Geometry: final body of the model. Coordinates: model frame, mm. A direction names the side the tool comes from. Give positions to 0.01 mm unless a question says otherwise; leave off trailing zeros. Write each loop counter-clockwise with the first axis right and the second up, starting at its lowest first coordinate (ties: lowest second). Pieces come first, ordered by that corner, then holes. Notation, with made-up numbers: (47, -36.5) -> (64, -36.5) arc R18 ccw to (64, -24.5) -> close; hole circle Ø6 at (32.5, 82.25). An arc over 180 degrees is marked (long way). Answer in a Markdown table with one row per item. Add a question column.
Item 1: Draft query along Z for faces 4 (the flat face through (350.266, 55, 187)), 5 (the flat face through (181.824, 28.354, 12.186)), 6 (the flat face through (182, 180, 0)), 7 (the flat face through (368.3, 213, 195)). Return one class per face: +Z half, -Z half, draft (parallel to the pull), parting line (faces both ways), or undercut.
Item 2: Section query B-B on y = 150. Output: boundary loops of the cut face in (x, z).
Item 3: Access query for faces 1 (the flat face through (181.824, 56.286, 19.184)), 2 (the flat face through (181.57, 397.83, 151.55)), 3 (the flat face through (181.82, 93.53, 364.05)). Directions: +Z, -Z, +X, -X, +Y, -Y. A direction counts if a zero-diameter tool reaches every point of the face in a straight line with its end or side. Return the directions, or none.
Item 4: First-contact query: P1, Ø5, axis at x = 274.5, z = 233, coming from the +Y side; P2, Ø8, axis at x = 277, z = 103, coming from the +Y side; P3, Ø1.5, axis at x = 294, y = 175, coming from the +Z side. Flat tips, straight axial feed; report the tip coordinate or a pass-through.
Item 5: Material intervals for probe 1 along X at (y, z) = (45, 133); probe 2 along Z at (x, y) = (68.5, 165); probe 3 along Z at (x, y) = (237.5, 21.5), sorted ascending. Write a range as from..to.
Item 6: Section query C-C on x = 191.5. Output: boundary loops of the cut face in (y, z).
Item 7: Section query A-A on x = 237. Output: boundary loops of the cut face in (y, z).
Item 8: Section query D-D on y = 296. Output: boundary loops of the cut face in (x, z), plus the area to 3 significant figures.
```python
from build123d import *

# Parameters (mm, degrees)
F1_DEPTH = 368.3
F2_W     = 332.232
F2_H     = 357.632
F3_DEPTH = 25.4
F4_R     = 130.175
F5_DEPTH = 10.16
F6_W     = 332.232
F6_H     = 25.4
F7_DEPTH = 25.4


with BuildPart() as f1:
    # F0 (on Right) → F1 (new body)
    with BuildSketch(Plane.YZ):
        Polygon((85.2122760074, 384.3677380031), (0, 0), (364.2337952902, 0), (432.3831361393, 307.4018112867), align=None)
    extrude(amount=F1_DEPTH)

    # F2 (on face) → F3 (cut)
    with BuildSketch(Plane(origin=(0, 0, 0), x_dir=(1, 0, 0), z_dir=(0, -0.9762960071, 0.2164396139))):
        with Locations((184.15, 196.85)):
            Rectangle(F2_W, F2_H)
    extrude(amount=-F3_DEPTH, mode=Mode.SUBTRACT)

    # F4 (on face) → F5 (join)
    with BuildSketch(Plane(origin=(0, 24.7979185808, -5.497566194), x_dir=(1, 0, 0), z_dir=(0, -0.9762960071, 0.2164396139))):
        with Locations((184.15, 210.566)):
            Circle(F4_R)
    extrude(amount=F5_DEPTH)

    # F6 (on face) → F7 (cut)
    with BuildSketch(Plane(origin=(0, 24.7979185808, -5.497566194), x_dir=(1, 0, 0), z_dir=(0, -0.9762960071, 0.2164396139))):
        with Locations((184.15, 30.734)):
            Rectangle(F6_W, F6_H)
    extrude(amount=-F7_DEPTH, mode=Mode.SUBTRACT)


solid = f1.part
```
Findings below:
| question | item | result |
|---|---|---|
| 1 | face 4 | undercut |
| 1 | face 5 | undercut |
| 1 | face 6 | -Z half |
| 1 | face 7 | draft |
| 2 | outline | (0, 0) -> (368.3, 0) -> (368.3, 370) -> (0, 370) -> close |
| 3 | face 1 | none |
| 3 | face 2 | -Z, +X, -X, +Y |
| 3 | face 3 | -Y |
| 4 | P1 | stops at y = 416.44 |
| 4 | P2 | stops at y = 387.96 |
| 4 | P3 | stops at z = 364.63 |
| 5 | probe 1 | x = 0..18.03, 350.27..368.3 |
| 5 | probe 2 | z = 0..366.68 |
| 5 | probe 3 | z = 0..13.71 |
| 6 | outline | (0, 0) -> (364.23, 0) -> (432.38, 307.4) -> (85.21, 384.37) -> (81.31, 366.76) -> (106.11, 361.26) -> (98.5, 326.96) -> (88.58, 329.16) -> (32.32, 75.39) -> (42.24, 73.19) -> (34.2, 36.91) -> (59, 31.41) -> (53.5, 6.61) -> (3.9, 17.61) -> close |
| 7 | outline | (0, 0) -> (364.23, 0) -> (432.38, 307.4) -> (85.21, 384.37) -> (81.31, 366.76) -> (106.11, 361.26) -> (96.12, 316.22) -> (86.2, 318.42) -> (34.71, 86.13) -> (44.62, 83.93) -> (34.2, 36.91) -> (59, 31.41) -> (53.5, 6.61) -> (3.9, 17.61) -> close |
| 8 | outline | (0, 0) -> (368.3, 0) -> (368.3, 337.64) -> (0, 337.64) -> close |
| 8 | area | 124,000 mm^2 |
